Input: part model. Units: mm. Frame: model coordinates. Face numbers are marked on the shaded views. A direction names the side the tool comes from. Round coordinates to 2 decimals unless told otherwise and drop trailing zeros. Loops run counter-clockwise (first coordinate to the right, second up) from the corner with the lowest first, then second, coordinate; pieces in that order, holes last.
(1) Cut plane D-D, the plane y = 37. Output: boundary loops of the cut face in (x, z).
(2) Access query for the marked faces 1, 2 and 3. Directions: +Z, -Z, +X, -X, +Y, -Y. A direction counts if a zero-diameter tool reaches every point of the face in a straight line with its end or side. Return the directions, or none.
(3) Cut plane A-A, the plane z = 10. Output: boundary loops of the cut face in (x, y), and give its area (3 significant figures).
(4) Cut plane B-B, the plane y = 25. Output: boundary loops of the cut face in (x, z), and give its area (3 significant figures).
(5) Line query: line 1 (Z direction, x = -26, y = 25); line 2 (Z direction, x = -16, y = 41); line 3 (X direction, y = 28, z = 31). Output: solid intervals per line, ascending.
(6) Cut plane C-C, the plane x = -20. Output: boundary loops of the cut face in (y, z).
(7) First-contact query: pin 1 Ø2 at (x, y) = (-9, 33) entering from +Z; pin 2 Ø1.5 at (y, z) = (20, 48.5) entering from -X; pin 3 Ø12 at (x, z) = (-5.5, 20) entering from -Y. Flat tips, straight axial feed; report the tip coordinate or a pass-through.
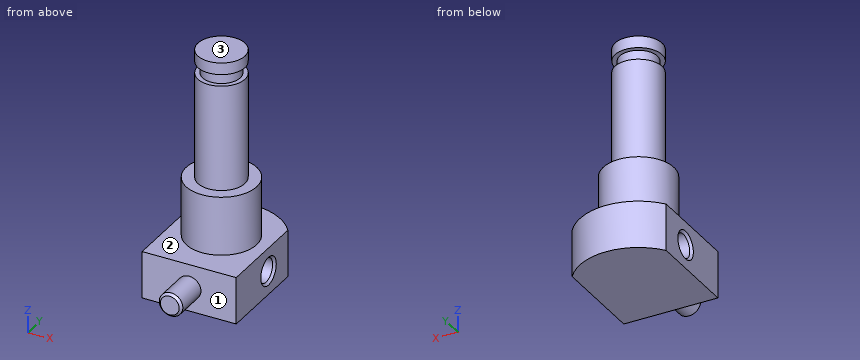
from build123d import *

# Parameters (mm, degrees)
F1_DEPTH  = 20
F2_R      = 5
F3_DEPTH  = 15
F4_R      = 15
F5_DEPTH  = 25
F6_R      = 10
F7_DEPTH  = 45
F8_R      = 8
F9_DEPTH  = 5
F10_R     = 10
F10_R_2   = 8
F11_DEPTH = 5
F12_R     = 5
F13_DEPTH = 45
F14_SIZE  = 1


with BuildPart() as f1:
    # F0 (on Top) → F1 (new body)
    with BuildSketch(Plane.XY):
        with BuildLine():
            Line((-40, 0), (0, 0))
            Line((0, 0), (0, 40))
            ThreePointArc((0, 40), (-20, 50), (-40, 40))
            Line((-40, 40), (-40, 0))
        make_face()
    extrude(amount=F1_DEPTH)

    # F2 (on face) → F3 (join)
    with BuildSketch(Plane.XZ):
        with Locations((-20, 10)):
            Circle(F2_R)
    extrude(amount=F3_DEPTH)

    # F4 (on face) → F5 (join)
    with BuildSketch(Plane.XY.offset(20)):
        with Locations((-20, 25)):
            Circle(F4_R)
    extrude(amount=F5_DEPTH)

    # F6 (on face) → F7 (join)
    with BuildSketch(Plane.XY.offset(45)):
        with Locations((-20, 25)):
            Circle(F6_R)
    extrude(amount=F7_DEPTH)

    # F8 (on face) → F9 (join)
    with BuildSketch(Plane.XY.offset(90)):
        with Locations((-20, 25)):
            Circle(F8_R)
    extrude(amount=F9_DEPTH)

    # F10 (on face) → F11 (join)
    with BuildSketch(Plane.XY.offset(95)):
        with Locations((-20, 25)):
            Circle(F10_R)
        with Locations((-20, 25)):
            Circle(F10_R_2, mode=Mode.SUBTRACT)
        with Locations((-20, 25)):
            Circle(F10_R_2)
    extrude(amount=F11_DEPTH)

    # F12 (on face) → F13 (cut)
    with BuildSketch(Plane.YZ):
        with Locations((25, 10)):
            Circle(F12_R)
    extrude(amount=-F13_DEPTH, mode=Mode.SUBTRACT)

    # F14
    f14_edges = [f1.edges().sort_by_distance(p)[0] for p in [
        (-25, -15, 10),
        (0, 20, 10),
        (-40, 20, 10),
    ]]
    chamfer(f14_edges, length=F14_SIZE)


solid = f1.part
Reported:
1. outline: (-40, 0) - (0, 0) - (0, 20) - (-11, 20) - (-11, 45) - (-29, 45) - (-29, 20) - (-40, 20) - close
2. face 1: -Y
2. face 2: +Z
2. face 3: +Z, +X, -X, +Y, -Y
3. outline: (-40, 0) - (-25, 0) - (-25, -14) - (-24, -15) - (-16, -15) - (-15, -14) - (-15, 0) - (0, 0) - (0, 19) - (-1, 20) - (-39, 20) - (-40, 19) - close; (-40, 31) - (-39, 30) - (-1, 30) - (0, 31) - (0, 40) arc R25 ccw to (-40, 40) - close
3. area: 1,630 mm2
4. outline: (-40, 0) - (0, 0) - (0, 4) - (-1, 5) - (-39, 5) - (-40, 4) - close; (-40, 16) - (-39, 15) - (-1, 15) - (0, 16) - (0, 20) - (-5, 20) - (-5, 45) - (-10, 45) - (-10, 90) - (-12, 90) - (-12, 95) - (-10, 95) - (-10, 100) - (-30, 100) - (-30, 95) - (-28, 95) - (-28, 90) - (-30, 90) - (-30, 45) - (-35, 45) - (-35, 20) - (-40, 20) - close
4. area: 2,230 mm2
5. line 1: z = 0 to 5, 15 to 100
5. line 2: z = 0 to 20
5. line 3: x = -34.7 to -5.3
6. outline: (-15, 6) - (-14, 5) - (0, 5) - (0, 0) - (50, 0) - (50, 20) - (40, 20) - (40, 45) - (35, 45) - (35, 90) - (33, 90) - (33, 95) - (35, 95) - (35, 100) - (15, 100) - (15, 95) - (17, 95) - (17, 90) - (15, 90) - (15, 45) - (10, 45) - (10, 20) - (0, 20) - (0, 15) - (-14, 15) - (-15, 14) - close; hole circle Ø10 at (25, 10)
7. pin 1: stops at z = 45
7. pin 2: stops at x = -29.05
7. pin 3: stops at y = 0
